Autodesk Inventor part; units mm, degrees
ref_plane "YZ Plane" through (0, 0, 0) normal (1, 0, 0) x (0, 1, 0)
ref_plane "XZ Plane" through (0, 0, 0) normal (0, 1, 0) x (-1, 0, 0)
ref_plane "XY Plane" through (0, 0, 0) normal (0, 0, 1) x (1, 0, 0)
sketch "Sketch1" plane through (0, 0, 0) normal (0, 0, 1) x (1, 0, 0)
  circle A0 centre (0, 0) radius 2.25
  circle A1 centre (-19.75, 0) radius 2.25
  circle A2 centre (19.75, 0) radius 2.25
  line L0 (0, 13.6364) -> (0, -14.2241) construction
  line L1 (-36.2718, 0) -> (35.3009, 0) construction
  line L2 (-22.75, 3) -> (22.75, 3)
  line L3 (22.75, 3) -> (22.75, -3)
  line L4 (22.75, -3) -> (-22.75, -3)
  line L5 (-22.75, -3) -> (-22.75, 3)
  line L6 (-22.75, -3) -> (22.75, -3)
  line L7 (22.75, -3) -> (22.75, -13)
  line L8 (22.75, -13) -> (-22.75, -13)
  line L9 (-22.75, -13) -> (-22.75, -3)
  line L10 (-22.75, -13) -> (22.75, -13)
  line L11 (22.75, -13) -> (22.75, -14.5)
  line L12 (22.75, -14.5) -> (-22.75, -14.5)
  line L13 (-22.75, -14.5) -> (-22.75, -13)
  dimension "d0" = 4.5
  dimension "d1" = 4.5
  dimension "d2" = 4.5
  dimension "d5" = 3
  dimension "d6" = 3
  dimension "d7" = 3
  dimension "d8" = 3
  dimension "d9" = 10
  dimension "d10" = 1.5
  dimension "d20" = 22
  dimension "d21" = 22
extrude "Extrusion1" add sketch "Sketch1" along normal blind 1.5
extrude "Extrusion2" add sketch "Sketch1" along normal blind 13.5 contours L8 L11 L12 L13
sketch "Sketch2" plane through (-22.75, -13, 1.5) normal (0, 1, 0) x (1, 0, 0)
  line L0 (45.5, 0) -> (45.5, -12)
  line L1 (0, -12) -> (45.5, -12)
  line L2 (45.5, -12) -> (45.5, -13.5)
  line L3 (45.5, -13.5) -> (0, -13.5)
  line L4 (0, -13.5) -> (0, -12)
  point P0 (22.75, 1.5)
  dimension "d15" = 1.5
extrude "Extrusion3" add sketch "Sketch2" against normal blind 1.5
extrude "Extrusion4" add sketch "Sketch2" along normal blind 8
properties part number "TopClip"
Check sheet for the modelled part. Datum: model origin and axes. Units: mm. A direction names the side the tool comes from. Round coordinates to 2 decimals unless told otherwise and drop trailing zeros. Write each loop counter-clockwise with the first axis right and the second up, starting at its lowest first coordinate (ties: lowest second). Pieces come first, ordered by that corner, then holes. Notation, with made-up numbers: (29, 3) -> (36, 3) arc R17 cw to (36, 29) -> close; hole circle Ø2 at (52.5, -31). An arc over 180 degrees is marked (long way). Put each result on its own line as item: value.
(1) Sectioned sample at B-B (x = 19.75). Enter the section's corners in (y, z).
Values found:
outline: (-14.5, 0) -> (-2.25, 0) -> (-2.25, 1.5) -> (-13, 1.5) -> (-13, 13.5) -> (-5, 13.5) -> (-5, 15) -> (-14.5, 15) -> close; (2.25, 0) -> (3, 0) -> (3, 1.5) -> (2.25, 1.5) -> close
(2) Material ranges on line 1 (Y direction, x = -19.75, z = 0.85); line 2 (Z direction, x = -9.5, y = -9.25); line 3 (Z direction, x = -5, y = 1.75), recorded low to high.
Values found:
line 1: y = -14.5 to -2.25, 2.25 to 3
line 2: z = 0 to 1.5, 13.5 to 15
line 3: z = 0 to 1.5
(3) Sectioned sample at D-D (z = 14.25). Enter the section's corners in (x, y), plus the area to 3 significant figures.
Values found:
outline: (-22.75, -14.5) -> (22.75, -14.5) -> (22.75, -5) -> (-22.75, -5) -> close
area: 432 mm^2
(4) Tool access check on faces 4 (the face through (0, -5, 14)), 5 (the face through (0, -9, 13.5)), 6 (the face through (0, -10, 15)). Record the directions out of +Z, -Z, +X, -X, +Y, -Y that give a thin tool (end or side, any length) a straight path to the whole face; none if there is none.
Values found:
face 4: +Z, +X, -X, +Y
face 5: +X, -X, +Y
face 6: +Z, +X, -X, +Y, -Y
(5) Mould release check, pull along Y, two halves, no side actions. Record for faces 1 (the face through (-17.604, -0.676, 0.74)), 2 (the face through (0, 3, 1)), 3 (the face through (0, -14.5, 7)): released by +Y, released by -Y, zero draft, split by the parting line, or undercut.
Values found:
face 1: undercut
face 2: released by +Y
face 3: released by -Y
(6) Sectioned sample at C-C (y = -6.75). Enter the section's corners in (x, z), plus the area to 4 significant figures.
Values found:
outline: (-22.75, 0) -> (22.75, 0) -> (22.75, 1.5) -> (-22.75, 1.5) -> close; (-22.75, 13.5) -> (22.75, 13.5) -> (22.75, 15) -> (-22.75, 15) -> close
area: 136.5 mm^2
(7) Sectioned sample at A-A (y = 0). Enter the section's corners in (x, z).
Values found:
outline: (-22.75, 0) -> (-22, 0) -> (-22, 1.5) -> (-22.75, 1.5) -> close; (-17.5, 0) -> (-2.25, 0) -> (-2.25, 1.5) -> (-17.5, 1.5) -> close; (2.25, 0) -> (17.5, 0) -> (17.5, 1.5) -> (2.25, 1.5) -> close; (22, 0) -> (22.75, 0) -> (22.75, 1.5) -> (22, 1.5) -> close
(8) Go/stop test with flat-tipped pins: pin 1 Ø6 at (x, z) = (-7.5, 7.5) entering from +Y; pin 2 Ø2.5 at (x, y) = (-19.75, 0) entering from -Z; pin 3 Ø3 at (x, y) = (-15, -1) entering from +Z. Record where each tip stops, or that it passes through.
Values found:
pin 1: stops at y = -13
pin 2: passes through
pin 3: stops at z = 1.5
